Can you work these out from the drawing? Everything is in mm from the part's minimum corner. A direction names the side the tool comes from. Round coordinates to 2 decimals unless told otherwise and drop trailing zeros. Loops run counter-clockwise (first coordinate to the right, second up) from the corner with the lowest first, then second, coordinate; pieces in that order, holes last. Notation, with made-up numbers: (-37, -10) - (6, -10) arc R7 ccw to (6, -6) - close; hole circle Ø2 at (-12, -6.5). An arc over 180 degrees is marked (long way). Answer as a JSON object with one key per item and string values. Group by question number.
1) If I drill on line 1 along Y through (x, z) = (7, 11); line 2 along Z through (x, y) = (45, 26.5); line 3 along X through (y, z) = (26.5, 25), over which ranges is the centre line in solid material (lowest first)? Write a range as [from, to].
2) I want a section at B-B, the plane y = 7.5. Please give me the cut outline in (x, z), then the cut area to 3 significant figures.
3) I want a section at D-D, the plane z = 19.5. Please give me the cut outline in (x, y), then the cut area to 3 significant figures.
4) If we mould it in two halves opening along X, with no side actions, what happens to the marked faces 5, 6, 7 and 8? For each: pulls with the +X half, pulls with the -X half, needs draft (parallel to the pull), parting line crosses it, or undercut.
5) I want a section at C-C, the plane x = 7. Please give me the cut outline in (y, z), then the cut area to 3 significant figures.
6) Which directions (+Z, -Z, +X, -X, +Y, -Y) give clear straight access to the entire face, cutting with the end or side of a thin tool? Please do the marked faces 1, 2, 3 and 4.
7) Will these pins go through, and if not, where does the flat tip stop? P1, Ø9, axis at x = 39.5, z = 19, coming from the -Y side; P2, Ø8, axis at x = 14, y = 48.5, coming from the +Z side; P3, Ø8, axis at x = 30, y = 40, coming from the -Z side; P4, Ø5, axis at y = 28, z = 25.5, coming from the -X side.
8) I want a section at A-A, the plane z = 25. Please give me the cut outline in (x, y), then the cut area to 3 significant figures.
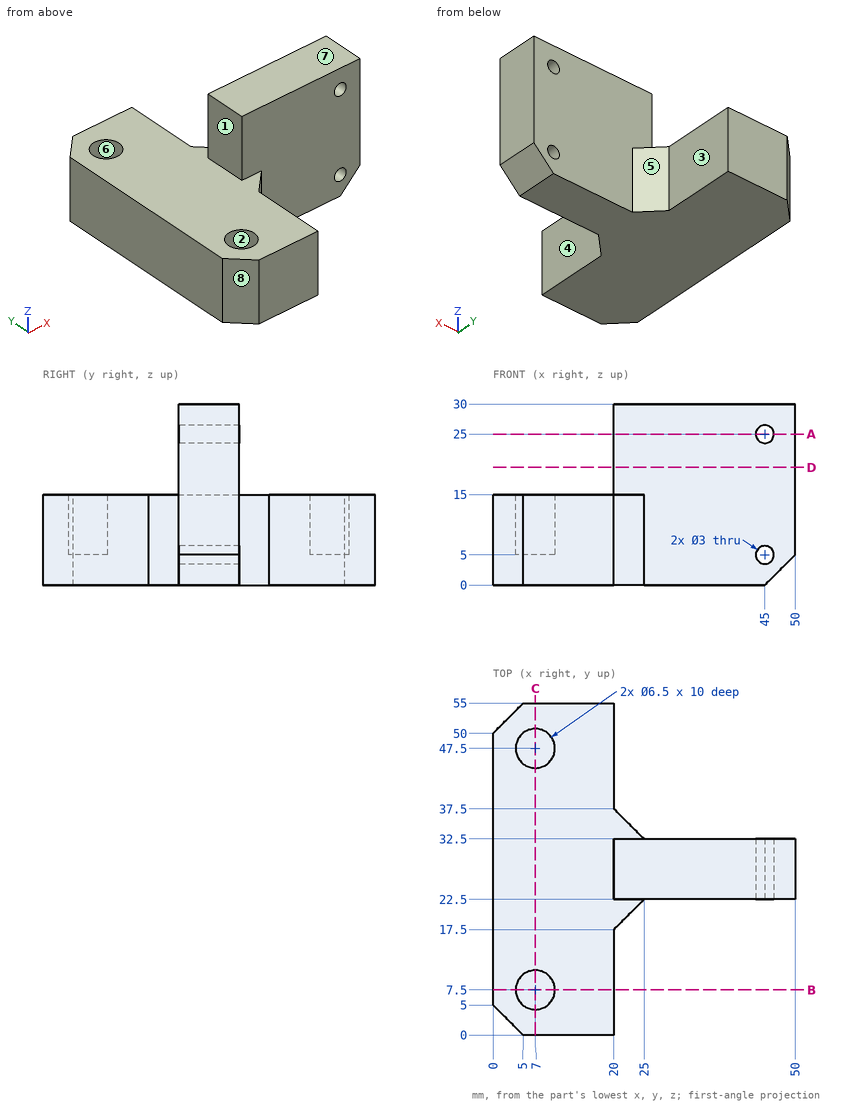
Outcome:
{
 "1": {"line 1": "[0, 4.25], [10.75, 44.25], [50.75, 55]", "line 2": "[0, 3.5], [6.5, 23.5], [26.5, 30]", "line 3": "[20, 43.5], [46.5, 50]"},
 "2": {"outline": "(0, 0) - (20, 0) - (20, 15) - (10.25, 15) - (10.25, 5) - (3.75, 5) - (3.75, 15) - (0, 15) - close", "area": "235 mm^2"},
 "3": {"outline": "(20, 22.5) - (50, 22.5) - (50, 32.5) - (20, 32.5) - close", "area": "300 mm^2"},
 "4": {"face 5": "pulls with the +X half", "face 6": "undercut", "face 7": "needs draft", "face 8": "pulls with the -X half"},
 "5": {"outline": "(0, 0) - (55, 0) - (55, 15) - (50.75, 15) - (50.75, 5) - (44.25, 5) - (44.25, 15) - (10.75, 15) - (10.75, 5) - (4.25, 5) - (4.25, 15) - (0, 15) - close", "area": "695 mm^2"},
 "6": {"face 1": "+Z, -X, +Y, -Y", "face 2": "+Z", "face 3": "+Z, -Z, +X, +Y", "face 4": "+Z, -Z, +X, -Y"},
 "7": {"P1": "y = 22.5", "P2": "z = 15", "P3": "through", "P4": "x = 20"},
 "8": {"outline": "(20, 22.5) - (43.5, 22.5) - (43.5, 32.5) - (20, 32.5) - close; (46.5, 22.5) - (50, 22.5) - (50, 32.5) - (46.5, 32.5) - close", "area": "270 mm^2"}
}
